For this review, take the finished solid that the model builds, in its own axes (mm). Face numbers are marked on the shaded views. A direction names the side the tool comes from. Coordinates: 2 decimals unless noted, no trailing zeros. Write each loop counter-clockwise with the first axis right and the second up, starting at its lowest first coordinate (ties: lowest second). Pieces come first, ordered by that corner, then holes. Notation, with made-up numbers: (65, 32) -> (114, 32) arc R16 cw to (114, 51) -> close; hole circle Ø10 at (31, 79.5). An arc over 180 degrees is marked (long way). One line per item, written item: value. Start each with the question number.
1) Mouldability with a two-part tool opening along Z and no side actions: class the marked faces 1, 2 and 3 as released by +Z, released by -Z, zero draft, split by the parting line, or undercut.
2) Add section A-A (z = -3.5). State the section outline as (x, y) points.
3) For probe 1 along Z at (x, y) = (4, 2.5); probe 2 along Y at (x, z) = (33.5, 10); probe 3 along X at (y, z) = (1.5, 22.5), list the stretches that pass through material, from the lowest coordinate up. Write a range as from..to.
4) Add section B-B (x = 30.5). State the section outline as (y, z) points.
5) For pin 1 Ø5.5 at (x, z) = (33, -6) entering from +Y; pin 2 Ø5 at (y, z) = (5, 7) entering from +X; pin 3 Ø1.5 at (x, y) = (15, 3.5) entering from -Z; pin 4 Ø1.5 at (x, z) = (8.5, -1.5) entering from -Y, all flat-tipped, find the tip position at first contact; note any pin that passes through.
6) Add section C-C (y = 1.25). State the section outline as (x, z) points, and give its area (3 significant figures).
7) Add section D-D (x = 6). State the section outline as (y, z) points, and give its area (3 significant figures).
8) Machinability: for the marked faces 4, 5 and 6, which of the approach directions +Z, -Z, +X, -X, +Y, -Y give a long, thin tool a straight path to every point of the face, cutting with its end or side? Answer none if there is none.
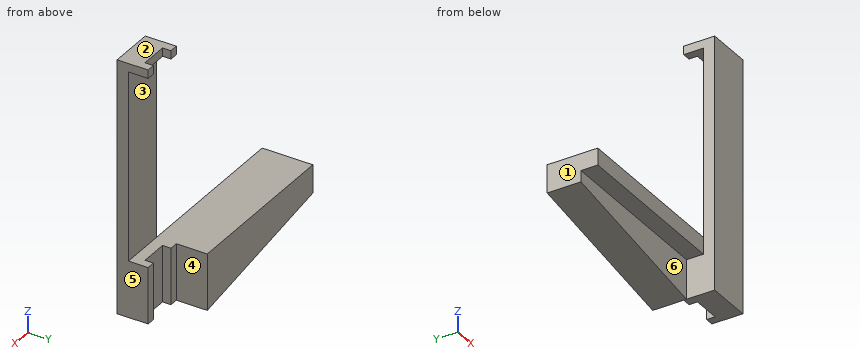
from build123d import *

# Parameters (mm, degrees)
BOSS_EXTRUDE1_DEPTH = 12
SKETCH2_W           = 8
SKETCH2_H           = 33.5
CUT_EXTRUDE1_DEPTH  = 10
SKETCH3_W           = 8
SKETCH3_H           = 45
CUT_EXTRUDE2_DEPTH  = 6.5
SKETCH4_W           = 5
SKETCH4_H           = 10
CUT_EXTRUDE3_DEPTH  = 1.5
SKETCH5_W           = 5
SKETCH5_H           = 1.5
CUT_EXTRUDE4_DEPTH  = 1.5
CUT_EXTRUDE5_DEPTH  = 2
CUT_EXTRUDE7_DEPTH  = 1
CUT_EXTRUDE9_DEPTH  = 3


with BuildPart() as part:
    # Sketch1 → Boss-Extrude1 (new body)
    with BuildSketch(Plane(origin=(0, 0, 0), x_dir=(1, 0, 0), z_dir=(0, 1, 0))):
        Polygon((0, 0), (30, 0), (30, -35), (38, -35), (38, 10), (30, 10), (0, 5), align=None)
    extrude(amount=BOSS_EXTRUDE1_DEPTH)

    # Sketch2 → Cut-Extrude1 (cut)
    with BuildSketch(Plane(origin=(0, 12, 0), x_dir=(1, 0, 0), z_dir=(0, 1, 0))):
        with Locations((34, -16.75)):
            Rectangle(SKETCH2_W, SKETCH2_H)
    extrude(amount=-CUT_EXTRUDE1_DEPTH, mode=Mode.SUBTRACT)

    # Sketch3 → Cut-Extrude2 (cut)
    with BuildSketch(Plane(origin=(0, 12, 0), x_dir=(1, 0, 0), z_dir=(0, 1, 0))):
        with Locations((34, -12.5)):
            Rectangle(SKETCH3_W, SKETCH3_H)
    extrude(amount=-CUT_EXTRUDE2_DEPTH, mode=Mode.SUBTRACT)

    # Sketch4 → Cut-Extrude3 (cut)
    with BuildSketch(Plane(origin=(0, 5.5, 0), x_dir=(1, 0, 0), z_dir=(0, 1, 0))):
        with Locations((34, 5)):
            Rectangle(SKETCH4_W, SKETCH4_H)
    extrude(amount=-CUT_EXTRUDE3_DEPTH, mode=Mode.SUBTRACT)

    # Sketch5 → Cut-Extrude4 (cut)
    with BuildSketch(Plane(origin=(0, 5.5, 0), x_dir=(1, 0, 0), z_dir=(0, 1, 0))):
        with Locations((34, -34.25)):
            Rectangle(SKETCH5_W, SKETCH5_H)
    extrude(amount=-CUT_EXTRUDE4_DEPTH, mode=Mode.SUBTRACT)

    # Sketch6 → Cut-Extrude5 (cut)
    with BuildSketch(Plane.XZ):
        Polygon((0, 0), (30, 0), (30, -10), (0, -5), align=None)
    extrude(amount=-CUT_EXTRUDE5_DEPTH, mode=Mode.SUBTRACT)

    # Sketch7 → Cut-Extrude7 (cut)
    with BuildSketch(Plane(origin=(0, 12, 0), x_dir=(1, 0, 0), z_dir=(0, 1, 0))):
        Polygon((0, 5), (30, 10), (30, 0), (0, 0), align=None)
    extrude(amount=-CUT_EXTRUDE7_DEPTH, mode=Mode.SUBTRACT)

    # Sketch10 → Cut-Extrude9 (cut)
    with BuildSketch(Plane.XZ.offset(-2)):
        Polygon((0, -5), (30, -10), (30, -3), (0, -3), align=None)
    extrude(amount=-CUT_EXTRUDE9_DEPTH, mode=Mode.SUBTRACT)


solid = part.part
Numbers:
1. face 1: zero draft
1. face 2: released by +Z
1. face 3: undercut
2. outline: (0, 5) -> (30, 5) -> (30, 0) -> (38, 0) -> (38, 5.5) -> (36.5, 5.5) -> (36.5, 4) -> (31.5, 4) -> (31.5, 5.5) -> (30, 5.5) -> (30, 11) -> (0, 11) -> close
3. probe 1: -3..0
3. probe 2: 0..2
3. probe 3: 30..38
4. outline: (0, -10) -> (5.5, -10) -> (5.5, 0) -> (2, 0) -> (2, 33.5) -> (5.5, 33.5) -> (5.5, 35) -> (0, 35) -> close
5. pin 1: y = 5.5
5. pin 2: through
5. pin 3: z = -3
5. pin 4: y = 2
6. outline: (30, -10) -> (38, -10) -> (38, 35) -> (30, 35) -> close
6. area: 360 mm²
7. outline: (2, -3) -> (5, -3) -> (5, -6) -> (11, -6) -> (11, 0) -> (2, 0) -> close
7. area: 45.0 mm²
8. face 4: +Z, -Z, +X, +Y
8. face 5: +Z, -Z, +X, +Y, -Y
8. face 6: -Z, -X, -Y
